The model under review builds one solid part; all positions refer to its coordinate system, in mm. A direction names the side the tool comes from. Round coordinates to 2 decimals unless told otherwise and drop trailing zeros. Loops run counter-clockwise (first coordinate to the right, second up) from the corner with the lowest first, then second, coordinate; pieces in that order, holes last. Notation, with made-up numbers: M 49,24.5 L 65,24.5 A27 ccw 65,54.5 Z; hole C 87.25,-21.75 d11. An arc over 180 degrees is marked long. Answer as a JSON object with one key per item and string values. Group by question number.
Item 1: Consider section C-C (z = 2.25). State how many separate pieces and enclosed holes the cut face has, and give its area (3 significant figures).
Item 2: To check wall thickness, follow line 1 (Y direction, x = 90, z = 1.9); line 2 (Y direction, x = 116, z = 2.65); line 3 (Y direction, x = 135, z = 0.9). State the ranges of each line that lie inside material, in increasing order.
Item 3: Tool access review of faces 1 (the face through (117.15, 183.01, 1.48)), 2 (the face through (89, 161, 3)): name each direction out of +Z, -Z, +X, -X, +Y, -Y from which nothing blocks a thin tool from reaching the whole face with its end or side.
Item 4: Consider section B-B (y = 129). Give the boundary of the cut face in (x, z).
Item 5: The part is to be moulded in two halves that separate along X. For faces 3 (the face through (74.404, 252.685, 1.479)), 4 (the face through (159.4, 79.49, 1.48)), 5 (the face through (2.85, 256.99, 1.48)), 6 (the face through (90.935, 0.008, 1.479)), say which applies: +X half, -X half, draft (parallel to the pull), parting line (faces both ways), or undercut.
Item 6: Consider section A-A (y = 165). Give the boundary of the cut face in (x, z), and give its area (3 significant figures).
Item 7: Insertion check: P1, Ø5, axis at x = 30, y = 221.5, coming from the -Z side; P2, Ø1, axis at x = 53, z = 1, coming from the -Y side; P3, Ø1.5, axis at x = 95.5, z = 1.5, coming from the -Y side; P4, Ø1.5, axis at y = 120, z = 0.5, coming from the -X side. Each pin has a flat end and moves straight along its axis. Give the tip position at first contact, or say it passes through.
Item 8: Consider section D-D (x = 159.5). Give the boundary of the cut face in (y, z).
Autodesk Fusion 360 part; units mm, degrees
sketch "Sketch1" plane through (0, 0, 0) normal (0, 0, 1) x (1, 0, 0)
  line L0 (180, 133.6216) -> (180, 250)
  line L1 (170, 260) -> (10, 260)
  line L2 (0, 250) -> (0, 133.4829)
  circle A0 centre (90.016, 55) radius 38
  circle A1 centre (90.016, 55) radius 42 construction
  circle A2 centre (30, 165) radius 2.75
  circle A3 centre (30, 221.5) radius 2.75
  line L3 (2.627, 123.5637) -> (39.0941, 34.2163)
  line L4 (177.3504, 123.503) -> (140.9438, 34.2308)
  arc A4 (0, 133.4829) -> (2.627, 123.5637) centre (39.6611, 138.6792) ccw
  arc A5 (177.3504, 123.503) -> (180, 133.6216) centre (140.312, 138.6078) ccw
  arc A6 (10, 260) -> (0, 250) centre (10, 250) ccw
  arc A7 (180, 250) -> (170, 260) centre (170, 250) ccw
  arc A8 (39.0941, 34.2163) -> (140.9438, 34.2308) centre (90.016, 55) ccw
  circle A9 centre (90, 97) radius 2.25
  circle A10 centre (60.3062, 84.6872) radius 2.25
  circle A11 centre (48.016, 54.984) radius 2.25
  circle A12 centre (60.3288, 25.2902) radius 2.25
  circle A13 centre (90.032, 13) radius 2.25
  circle A14 centre (119.7258, 25.3128) radius 2.25
  circle A15 centre (132.016, 55.016) radius 2.25
  circle A16 centre (119.7032, 84.7098) radius 2.25
  circle A17 centre (150, 221.5) radius 2.75
  circle A18 centre (150, 165) radius 2.75
  circle A19 centre (61.75, 154) radius 2.75
  circle A20 centre (118.25, 154) radius 2.75
  line L5 (77.016, 104) -> (103.016, 104)
  line L6 (105.016, 106) -> (105.016, 112)
  line L7 (103.016, 114) -> (77.016, 114)
  line L8 (75.016, 112) -> (75.016, 106)
  arc A21 (77.016, 114) -> (75.016, 112) centre (77.016, 112) ccw
  arc A22 (75.016, 106) -> (77.016, 104) centre (77.016, 106) ccw
  arc A23 (103.016, 104) -> (105.016, 106) centre (103.016, 106) ccw
  arc A24 (105.016, 112) -> (103.016, 114) centre (103.016, 112) ccw
  circle A25 centre (15, 129) radius 2.75
  circle A26 centre (15, 250) radius 2.75
  circle A27 centre (45, 250) radius 2.75
  circle A28 centre (45, 129) radius 2.75
  circle A29 centre (75, 250) radius 2.75
  circle A30 centre (105, 250) radius 2.75
  circle A31 centre (135, 250) radius 2.75
  circle A32 centre (135, 129) radius 2.75
  circle A33 centre (165, 250) radius 2.75
  circle A34 centre (165, 129) radius 2.75
  line L9 (110, 180) -> (70, 180)
  line L10 (60, 190) -> (60, 220)
  line L11 (70, 230) -> (110, 230)
  line L12 (120, 220) -> (120, 190)
  arc A35 (70, 230) -> (60, 220) centre (70, 220) ccw
  arc A36 (120, 220) -> (110, 230) centre (110, 220) ccw
  arc A37 (110, 180) -> (120, 190) centre (110, 190) ccw
  arc A38 (60, 190) -> (70, 180) centre (70, 190) ccw
  circle A39 centre (75, 129) radius 2.75
  circle A40 centre (105, 129) radius 2.75
  point P0 (180, 260)
  point P1 (0, 260)
  point P2 (0, 130)
  point P3 (75.016, 104)
  point P4 (105.016, 114)
  point P5 (75.016, 114)
  dimension "d1" = 260
  dimension "d3" = 76
  dimension "d4" = 84
  dimension "d5" = 110
  dimension "d8" = 130
  dimension "d9" = 180
  dimension "d10" = 40
  dimension "d11" = 10
  dimension "d12" = 4.5
  dimension "d13" = 90
  dimension "d15" = 360
  dimension "d16" = 5.5
  dimension "d17" = 5.5
  dimension "d18" = 56.5
  dimension "d19" = 110
  dimension "d22" = 120
  dimension "d23" = 0
  dimension "d24" = 30
  dimension "d25" = 30
  dimension "d26" = 5.5
  dimension "d27" = 5.5
  dimension "d28" = 56.5
  dimension "d29" = 61.75
  dimension "d32" = 30
  dimension "d33" = 10
  dimension "d34" = 15
  dimension "d35" = 49
  dimension "d36" = 2
  dimension "d37" = 5.5
  dimension "d38" = 15
  dimension "d39" = 5.5
  dimension "d40" = 15
  dimension "d41" = 10
  dimension "d44" = 30
  dimension "d45" = 0
  dimension "d46" = 60
  dimension "d47" = 60
  dimension "d48" = 50
  dimension "d49" = 30
  dimension "d50" = 10
  dimension "d54" = 40
  dimension "d57" = 15
  dimension "d60" = 60
  dimension "d61" = 0
extrude "Extrude1" add sketch "Sketch1" along normal blind 3
extrude "Extrude3" cut sketch "Sketch1" along normal through all contours A39 | A40
extrude "Extrude2" [suppressed]
equation "d29 = ( ( 180 - 56.5 ) / 2 ) * 1 mm"
Geometry results:
{
 "1": {"separate pieces": "1", "enclosed holes": "29", "area": "31,100 mm^2"},
 "2": {"line 1": "y = 0 to 10.75, 15.25 to 17, 93 to 94.75, 99.25 to 104, 114 to 180, 230 to 260", "line 2": "y = 6.52 to 27.27, 82.73 to 152.42, 155.58 to 182, 228 to 260", "line 3": "y = 23.35 to 126.25, 131.75 to 247.25, 252.75 to 260"},
 "3": {"face 1": "+Z, -Z", "face 2": "+Z, +X, -X, +Y, -Y"},
 "4": {"outline": "M 0.85,0 L 12.25,0 L 12.25,3 L 0.85,3 Z; M 17.75,0 L 42.25,0 L 42.25,3 L 17.75,3 Z; M 47.75,0 L 72.25,0 L 72.25,3 L 47.75,3 Z; M 77.75,0 L 102.25,0 L 102.25,3 L 77.75,3 Z; M 107.75,0 L 132.25,0 L 132.25,3 L 107.75,3 Z; M 137.75,0 L 162.25,0 L 162.25,3 L 137.75,3 Z; M 167.75,0 L 179.14,0 L 179.14,3 L 167.75,3 Z"},
 "5": {"face 3": "undercut", "face 4": "+X half", "face 5": "-X half", "face 6": "parting line"},
 "6": {"outline": "M 0,0 L 27.25,0 L 27.25,3 L 0,3 Z; M 32.75,0 L 147.25,0 L 147.25,3 L 32.75,3 Z; M 152.75,0 L 180,0 L 180,3 L 152.75,3 Z", "area": "507 mm^2"},
 "7": {"P1": "passes through", "P2": "stops at y = 13.87", "P3": "stops at y = 0.2", "P4": "stops at x = 3.78"},
 "8": {"outline": "M 79.73,0 L 260,0 L 260,3 L 79.73,3 Z"}
}
